```python
from build123d import *

# Parameters (mm, degrees)
SKETCH2_R           = 1.699999062
SKETCH2_R_2         = 1.69999994
BOSS_EXTRUDE1_DEPTH = 4
BOSS_EXTRUDE2_DEPTH = 8
SKETCH4_R           = 1.7
CUT_EXTRUDE1_DEPTH  = 93


# Read off the part's stored shape, not the designer's step: Surface-Imported1
with BuildPart() as part:
    # Sketch2 → Boss-Extrude1 (new body)
    with BuildSketch(Plane(origin=(0, 0, 0), x_dir=(1, 0, 0), z_dir=(0, 1, 0))):
        with BuildLine():
            Line((6.000000983, 0), (52.999999374, 0))
            ThreePointArc((52.999999374, 0), (57.242640757, -1.757359601), (59.000000358, -6.000000983))
            Line((59.000000358, -6.000000983), (59.000000358, -63.999995589))
            ThreePointArc((59.000000358, -63.999995589), (57.242641528, -68.242638834), (52.999999374, -70.000000298))
            Line((52.999999374, -70.000000298), (6.000000983, -70.000000298))
            ThreePointArc((6.000000983, -70.000000298), (1.75735699, -68.242640674), (0, -63.999995589))
            Line((0, -63.999995589), (0, -6.000000983))
            ThreePointArc((0, -6.000000983), (1.757359601, -1.757359601), (6.000000983, 0))
        make_face()
        with Locations(Location((12.000001036, -10.99999994, 0), (0, 0, 270))):
            Circle(SKETCH2_R, mode=Mode.SUBTRACT)
        with Locations(Location((22.000001036, -10.99999994, 0), (0, 0, 270))):
            Circle(SKETCH2_R, mode=Mode.SUBTRACT)
        with Locations(Location((22.000001036, -59.000000715, 0), (0, 0, 270))):
            Circle(SKETCH2_R, mode=Mode.SUBTRACT)
        with Locations(Location((12.000001036, -59.000000715, 0), (0, 0, 270))):
            Circle(SKETCH2_R, mode=Mode.SUBTRACT)
        with Locations(Location((41.50000118, -27.999999899, 0), (0, 0, 270))):
            Circle(SKETCH2_R_2, mode=Mode.SUBTRACT)
        with Locations(Location((41.50000118, -43.499999899, 0), (0, 0, 270))):
            Circle(SKETCH2_R_2, mode=Mode.SUBTRACT)
        with BuildLine():
            Line((32.499998808, -46.500001103), (32.499998808, -25.499999523))
            ThreePointArc((32.499998808, -25.499999523), (32.207106087, -24.792893943), (31.500000507, -24.500001222))
            Line((31.500000507, -24.500001222), (28.500001878, -24.500001222))
            ThreePointArc((28.500001878, -24.500001222), (27.792893663, -24.20710741), (27.499999851, -23.499999195))
            Line((27.499999851, -23.499999195), (27.499999851, -14.499999583))
            Line((27.499999851, -14.499999583), (6.500001065, -14.499999583))
            Line((6.500001065, -14.499999583), (6.500001065, -55.500000715))
            Line((6.500001065, -55.500000715), (27.499999851, -55.500000715))
            Line((27.499999851, -55.500000715), (27.499999851, -48.500001431))
            ThreePointArc((27.499999851, -48.500001431), (27.792894046, -47.792893599), (28.500001878, -47.499999404))
            Line((28.500001878, -47.499999404), (31.500000507, -47.499999404))
            ThreePointArc((31.500000507, -47.499999404), (32.207106087, -47.207106683), (32.499998808, -46.500001103))
        make_face(mode=Mode.SUBTRACT)
        with BuildLine():
            Line((34.55240652, -51.235973835), (44.55240652, -51.235973835))
            ThreePointArc((44.55240652, -51.235973835), (45.259513765, -51.528867517), (45.55240652, -52.235975146))
            Line((45.55240652, -52.235975146), (45.55240652, -58.235975146))
            ThreePointArc((45.55240652, -58.235975146), (45.259513301, -58.943081927), (44.55240652, -59.235975146))
            Line((44.55240652, -59.235975146), (34.55240652, -59.235975146))
            ThreePointArc((34.55240652, -59.235975146), (33.845298305, -58.943081334), (33.552404493, -58.23597312))
            Line((33.552404493, -58.23597312), (33.552404493, -52.235975862))
            ThreePointArc((33.552404493, -52.235975862), (33.845297712, -51.528867054), (34.55240652, -51.235973835))
        make_face(mode=Mode.SUBTRACT)
    extrude(amount=BOSS_EXTRUDE1_DEPTH)

    # Sketch3 → Boss-Extrude2 (add)
    with BuildSketch(Plane(origin=(0, 4, 0), x_dir=(1, 0, 0), z_dir=(0, 1, 0))):
        with BuildLine():
            Line((2, -7), (2, -63.000000298))
            ThreePointArc((2, -63.000000298), (3.464466094, -66.535534204), (7, -68.000000298))
            Line((7, -68.000000298), (52.000000358, -68.000000298))
            ThreePointArc((52.000000358, -68.000000298), (55.535534264, -66.535534204), (57.000000358, -63.000000298))
            Line((57.000000358, -63.000000298), (57.000000358, -7))
            ThreePointArc((57.000000358, -7), (55.535534264, -3.464466094), (52.000000358, -2))
            Line((52.000000358, -2), (7, -2))
            ThreePointArc((7, -2), (3.464466094, -3.464466094), (2, -7))
        make_face()
        with BuildLine():
            Line((4.8, -7), (4.8, -63.000000298))
            ThreePointArc((4.8, -63.000000298), (5.444365081, -64.555635217), (7, -65.200000298))
            Line((7, -65.200000298), (52.000000358, -65.200000298))
            ThreePointArc((52.000000358, -65.200000298), (53.555635276, -64.555635217), (54.200000358, -63.000000298))
            Line((54.200000358, -63.000000298), (54.200000358, -7))
            ThreePointArc((54.200000358, -7), (53.555635276, -5.444365081), (52.000000358, -4.8))
            Line((52.000000358, -4.8), (7, -4.8))
            ThreePointArc((7, -4.8), (5.444365081, -5.444365081), (4.8, -7))
        make_face(mode=Mode.SUBTRACT)
    extrude(amount=BOSS_EXTRUDE2_DEPTH)

    # Sketch4 → Cut-Extrude1 (cut)
    with BuildSketch(Plane(origin=(57.000000358, 0, 0), x_dir=(0, 0, -1), z_dir=(1, 0, 0))):
        with Locations((-34.000000298, 8)):
            Circle(SKETCH4_R)
    extrude(amount=-CUT_EXTRUDE1_DEPTH, mode=Mode.SUBTRACT)


solid = part.part
```
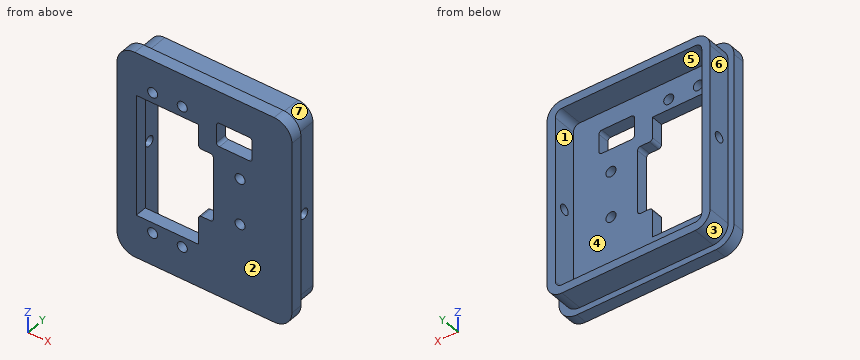
Design review of the part built by this model. Coordinates are the model's own, in mm. Face numbers are marked on the shaded views. A direction names the side the tool comes from. Give positions to 0.01 mm unless a question says otherwise; leave off trailing zeros. Order: outer loops, then holes, each group sorted by start corner. A loop starts at its lowest first (then second) coordinate and runs counter-clockwise, first axis right, second up. Notation, with made-up numbers: (58, 43) -> (85, 43) arc R20 ccw to (85, 49) -> close; hole circle Ø7 at (-32.75, 41). An arc over 180 degrees is marked (long way). Write item = value, one per line. Start each with the question number.
(1) For the marked faces 5, 6 and 7, list the 3-axis set-ups (+Z, -Z, +X, -X, +Y, -Y) from which the entire face can be reached by the end or side of a thin tool; tool diameter is ignored.
(2) To check wall thickness, follow line 1 along X through (y, z) = (2.25, 11); line 2 along X through (y, z) = (11.25, 11); line 3 along Z through (x, y) = (44.5, 5.5). State the ranges of each line that lie inside material, in increasing order.
(3) Mouldability with a two-part tool opening along Z and no side actions: class the marked faces 1, 2, 3 and 4 as +Z half, -Z half, draft (parallel to the pull), parting line (faces both ways), or undercut.
(4) We need section D-D on z = 43.5. Write out the cut boundary in (x, y), plus the area to 3 significant figures.
(5) For pin 1 (3 mm diameter, centred on x = 12, z = 59, fed in from -Y); pin 2 (15 mm diameter, centred on x = 38, z = 43, fed in from +Y); pin 3 (2.5 mm diameter, centred on x = 34, y = 6.5, fed in from -Z); pin 4 (1.5 mm diameter, centred on y = 7.5, z = 16.5, fed in from +X), all flat-tipped, find the tip position at first contact; note any pin that passes through.
(6) We need section C-C on y = 8. Write out the cut boundary in (x, z), plus the area to 3 significant figures.
(7) We need section B-B on x = 29.5. Write out the cut boundary in (y, z), plus the area to 3 significant figures.
(8) We need section A-A on z = 34. Write out the cut boundary in (x, y), plus the area to 3 significant figures.
Numbers:
q1.face_5 = +Y
q1.face_6 = +Z, -Z, -X, +Y
q1.face_7 = +Z, +X, +Y
q2.line_1 = 0 to 10.3, 13.7 to 20.3, 23.7 to 59
q2.line_2 = 2 to 4.8, 54.2 to 57
q2.line_3 = 2 to 4.8, 65.2 to 68
q3.face_1 = undercut
q3.face_2 = draft
q3.face_3 = -Z half
q3.face_4 = undercut
q4.outline = (0, 0) -> (6.5, 0) -> (6.5, 4) -> (4.8, 4) -> (4.8, 12) -> (2, 12) -> (2, 4) -> (0, 4) -> close; (32.5, 0) -> (39.8, 0) -> (39.8, 4) -> (32.5, 4) -> close; (43.2, 0) -> (59, 0) -> (59, 4) -> (57, 4) -> (57, 12) -> (54.2, 12) -> (54.2, 4) -> (43.2, 4) -> close
q4.area = 163 mm^2
q5.pin_1 = through
q5.pin_2 = 4
q5.pin_3 = 2
q5.pin_4 = 57
q6.outline = (2, 7) arc R5 ccw to (7, 2) -> (52, 2) arc R5 ccw to (57, 7) -> (57, 32.3) -> (54.2, 32.3) -> (54.2, 7) arc R2.2 cw to (52, 4.8) -> (7, 4.8) arc R2.2 cw to (4.8, 7) -> (4.8, 32.3) -> (2, 32.3) -> close; (2, 35.7) -> (4.8, 35.7) -> (4.8, 63) arc R2.2 cw to (7, 65.2) -> (52, 65.2) arc R2.2 cw to (54.2, 63) -> (54.2, 35.7) -> (57, 35.7) -> (57, 63) arc R5 ccw to (52, 68) -> (7, 68) arc R5 ccw to (2, 63) -> close
q6.area = 610 mm^2
q7.outline = (0, 0) -> (4, 0) -> (4, 2) -> (12, 2) -> (12, 4.8) -> (4, 4.8) -> (4, 24.5) -> (0, 24.5) -> close; (0, 47.5) -> (4, 47.5) -> (4, 65.2) -> (12, 65.2) -> (12, 68) -> (4, 68) -> (4, 70) -> (0, 70) -> close
q7.area = 233 mm^2
q8.outline = (0, 0) -> (6.5, 0) -> (6.5, 4) -> (4.8, 4) -> (4.8, 6.3) -> (2, 6.3) -> (2, 4) -> (0, 4) -> close; (2, 9.7) -> (4.8, 9.7) -> (4.8, 12) -> (2, 12) -> close; (32.5, 0) -> (59, 0) -> (59, 4) -> (57, 4) -> (57, 6.3) -> (54.2, 6.3) -> (54.2, 4) -> (32.5, 4) -> close; (54.2, 9.7) -> (57, 9.7) -> (57, 12) -> (54.2, 12) -> close
q8.area = 158 mm^2
